Read the model definition and answer for the solid it produces. Units are mm, in the model's axes. A direction names the side the tool comes from. Coordinates: 2 decimals unless noted, no trailing zeros. Loops run counter-clockwise (first coordinate to the right, second up) from the corner with the lowest first, then second, coordinate; pieces in that order, holes last. Notation, with made-up numbers: (15, 71.5) -> (33, 71.5) arc R15 cw to (33, 80.5) -> close; hole circle Ø1 at (34, 6.25). An arc over 180 degrees is marked (long way). Answer as CSV lines item,"result".
```python
from build123d import *

# Parameters (mm, degrees)
F0_W     = 19.05
F0_H     = 166.624
F1_DEPTH = 206.375
F2_W     = 22.225
F2_H     = 20.828
F3_DEPTH = 19.051
F5_W     = 9.525
F5_H     = 15.875
F6_DEPTH = 412.751
F8_R     = 101.6
F9_DEPTH = 10.4902


with BuildPart() as f1:
    # F0 (on Front) → F1 (new body)
    with BuildSketch(Plane.XZ):
        with Locations((-9.525, 83.312)):
            Rectangle(F0_W, F0_H)
    extrude(amount=-F1_DEPTH)

    # F2 (on Right) → F3 (cut, through all)
    with BuildSketch(Plane.YZ):
        with Locations((11.1125, 31.242)):
            Rectangle(F2_W, F2_H)
        with Locations((11.1125, 72.898)):
            Rectangle(F2_W, F2_H)
        with Locations((11.1125, 114.554)):
            Rectangle(F2_W, F2_H)
        with Locations((11.1125, 156.21)):
            Rectangle(F2_W, F2_H)
    extrude(amount=-F3_DEPTH, mode=Mode.SUBTRACT)

    # F4: F1 across face


with BuildPart() as f1_1:
    add(f1.part)
    add(f1.part.mirror(Plane(origin=(-9.525, 206.375, 83.312), x_dir=(1, 0, 0), z_dir=(0, 1, 0))))

    # F5 (on Front) → F6 (cut, through all)
    with BuildSketch(Plane.XZ):
        with Locations((-4.7625, 158.6865)):
            Rectangle(F5_W, F5_H)
    extrude(amount=-F6_DEPTH, mode=Mode.SUBTRACT)

    # F8 (on offset) → F9 (cut, symmetric)
    with BuildSketch(Plane.XY.offset(76.2)):
        with Locations((-111.125, 195.2625)):
            Circle(F8_R)
    extrude(amount=F9_DEPTH, both=True, mode=Mode.SUBTRACT)


solid = f1_1.part
```
Q1. For a pull along X with two mould halves and no side action, classify faces 6 (the face through (0, 209, 74)), 7 (the face through (-9, 402, 62.484)) as pulls with the +X half, pulls with the -X half, needs draft (parallel to the pull), parting line crosses it, or undercut.
Results:
face 6,"pulls with the +X half"
face 7,"needs draft"
Q2. Find the intervals of material crossed by probe 1 along Z at (x, y) = (-15, 212.5); probe 2 along Y at (x, z) = (-3.25, 82) (3 decimals); probe 3 along Z at (x, y) = (-2.25, 112), in increasing order. Write a range as [from, to].
Results:
probe 1,"z = [0, 65.71], [86.69, 166.62]"
probe 2,"y = [22.225, 390.525]"
probe 3,"z = [0, 150.75]"
Q3. For faces 1 (the face through (-9, 11, 20.828)), 2 (the face through (-5, 204, 150.749)), 3 (the face through (-15, 196, 65.71)), 4 (the face through (-14, 22.225, 154)), 5 (the face through (-9, 402, 41.656)), determine the directions among +Z, -Z, +X, -X, +Y, -Y from which every point of the face is accessible in a straight line to the end or side of a thin tool.
Results:
face 1,"+X, -X, -Y"
face 2,"+Z, +X, +Y, -Y"
face 3,"-X"
face 4,"+Z, +X, -X, -Y"
face 5,"+X, -X, +Y"
Q4. A cutting plane is placed at C-C, the plane z = 108.5. Write down the section's boundary in (x, y) (3 decimals), and give its area (3 significant figures).
Results:
outline,"(-19.05, 22.225) -> (0, 22.225) -> (0, 390.525) -> (-19.05, 390.525) -> close"
area,"7,020 mm²"
Q5. A cutting plane is placed at B-B, the plane y = 215.5. Write down the section's boundary in (x, z) (3 decimals).
Results:
outline,"(-19.05, 0) -> (0, 0) -> (0, 150.749) -> (-9.525, 150.749) -> (-9.525, 166.624) -> (-19.05, 166.624) -> (-19.05, 86.69) -> (-11.561, 86.69) -> (-11.561, 65.71) -> (-19.05, 65.71) -> close"
Q6. Given pin 1 Ø5 at (x, y) = (-5.5, 120.5) entering from +Z; pin 2 Ø9.5 at (x, y) = (-6.5, 6) entering from +Z; pin 3 Ø9.5 at (x, z) = (-11.5, 111.5) entering from +Y (3 decimals), each flat-ended and moving along its own axis, determine where each tip first touches the part or whether it passes through.
Results:
pin 1,"stops at z = 150.75"
pin 2,"stops at z = 145.8"
pin 3,"stops at y = 390.525"
